Part model, mm, in its own coordinate system. Coordinates: 2 decimals unless noted, no trailing zeros. Loops run counter-clockwise (first coordinate to the right, second up) from the corner with the lowest first, then second, coordinate; pieces in that order, holes last. Notation, with made-up numbers: M -2.75,83 L 10.25,83 A21 ccw 10.25,120 Z; hole C -36,69.25 d5. An arc over 180 degrees is marked long. Answer as CSV lines item,"result". Start each with the question number.
from build123d import *

# Parameters (mm, degrees)
SKETCH1_W           = 57.15
SKETCH1_H           = 25.4
SKETCH1_R           = 2.5527
BOSS_EXTRUDE1_DEPTH = 3.175
FILLET1_R           = 6.35


with BuildPart() as part:
    # Sketch1 → Boss-Extrude1 (new body)
    with BuildSketch(Plane.XY):
        with Locations((28.575, -12.7)):
            Rectangle(SKETCH1_W, SKETCH1_H)
        with Locations((12.7, -12.7)):
            Circle(SKETCH1_R, mode=Mode.SUBTRACT)
        with Locations((38.1, -12.7)):
            Circle(SKETCH1_R, mode=Mode.SUBTRACT)
        with Locations((47.625, -12.7)):
            Circle(SKETCH1_R, mode=Mode.SUBTRACT)
    extrude(amount=BOSS_EXTRUDE1_DEPTH)

    # Fillet1
    fillet1_edges = [part.edges().sort_by_distance(p)[0] for p in [
        (0, 0, 1.5875),
        (57.15, 0, 1.5875),
        (57.15, -25.4, 1.5875),
        (0, -25.4, 1.5875),
    ]]
    fillet(fillet1_edges, radius=FILLET1_R)


solid = part.part
Q1. Two-plate mould, pull along X, no slides. Class faces 1 (the face through (45.599, -14.253, 1.565)), 2 (the face through (28, 0, 2)), 3 (the face through (57.15, -13, 2)), 4 (the face through (15.058, -13.678, 1.565)): +X half, -X half, draft (parallel to the pull), parting line (faces both ways), or undercut.
Q2. Wall check: L1, parallel to Y at x = 12.7, z = 2.2; L2, parallel to Y at x = 49, z = 1.95; L3, parallel to X at y = -12, z = 0.4. Give the ranges that are in metal, low to high.
Q3. Slice it at D-D, the plane y = -2.5. Write the cut outline in (x, z) (3 decimals).
Q4. Flat gauge pin, fed straight in: P1, Ø5, axis at x = 31.5, y = -12, coming from the -Z side. Where does the tip first touch, or does it go through?
Q5. Slice it at C-C, the plane z = 0.65. Write the cut outline in (x, y) (3 decimals).
Q6. Slice it at A-A, the plane y = -12.7. Write the cut outline in (x, z) (3 decimals), and give its area (3 significant figures).
Q7. Slice it at B-B, the plane x = 38.1. Write the cut outline in (y, z) (3 decimals).
Solved:
1,face 1,"undercut"
1,face 2,"draft"
1,face 3,"+X half"
1,face 4,"undercut"
2,L1,"y = -25.4 to -15.25, -10.15 to 0"
2,L2,"y = -25.4 to -14.85, -10.55 to 0"
2,L3,"x = 0 to 10.25, 15.15 to 35.65, 40.55 to 45.17, 50.08 to 57.15"
3,outline,"M 1.3,0 L 55.85,0 L 55.85,3.175 L 1.3,3.175 Z"
4,P1,"stops at z = 0"
5,outline,"M 0,-19.05 A6.35 ccw 6.35,-25.4 L 50.8,-25.4 A6.35 ccw 57.15,-19.05 L 57.15,-6.35 A6.35 ccw 50.8,0 L 6.35,0 A6.35 ccw 0,-6.35 Z; hole C 12.7,-12.7 d5.105; hole C 38.1,-12.7 d5.105; hole C 47.625,-12.7 d5.105"
6,outline,"M 0,0 L 10.147,0 L 10.147,3.175 L 0,3.175 Z; M 15.253,0 L 35.547,0 L 35.547,3.175 L 15.253,3.175 Z; M 40.653,0 L 45.072,0 L 45.072,3.175 L 40.653,3.175 Z; M 50.178,0 L 57.15,0 L 57.15,3.175 L 50.178,3.175 Z"
6,area,"133 mm2"
7,outline,"M -25.4,0 L -15.253,0 L -15.253,3.175 L -25.4,3.175 Z; M -10.147,0 L 0,0 L 0,3.175 L -10.147,3.175 Z"
